from build123d import *

# Parameters (mm, degrees)
F0_W     = 70
F0_H     = 7
F1_DEPTH = 3
F2_R     = 3.49999


# Not quite as in the source:
# - a fillet or chamfer is up to 0.001 mm smaller than in the source, because OpenCascade refuses the exact size


with BuildPart() as f1:
    # F0 (on Top) → F1 (new body)
    with BuildSketch(Plane.XY):
        Rectangle(F0_W, F0_H)
        with BuildLine():
            Line((-20, -1.6), (-30, -1.6))
            ThreePointArc((-30, -1.6), (-31.6, 0), (-30, 1.6))
            Line((-30, 1.6), (-20, 1.6))
            ThreePointArc((-20, 1.6), (-18.4, 0), (-20, -1.6))
        make_face(mode=Mode.SUBTRACT)
        with BuildLine():
            Line((20, 1.6), (30, 1.6))
            ThreePointArc((30, 1.6), (31.6, 0), (30, -1.6))
            Line((30, -1.6), (20, -1.6))
            ThreePointArc((20, -1.6), (18.4, 0), (20, 1.6))
        make_face(mode=Mode.SUBTRACT)
    extrude(amount=F1_DEPTH)

    # F2 (radius 3.5 in the source; OpenCascade refuses exactly that, so slightly less here)
    f2_edges = [f1.edges().sort_by_distance(p)[0] for p in [
        (-35, 3.5, 1.5),
        (-35, -3.5, 1.5),
        (35, 3.5, 1.5),
        (35, -3.5, 1.5),
    ]]
    fillet(f2_edges, radius=F2_R)


solid = f1.part
Verification items for the finished model (mm, model axes). A direction names the side the tool comes from. Coordinates: 2 decimals unless noted, no trailing zeros. Loops run counter-clockwise (first coordinate to the right, second up) from the corner with the lowest first, then second, coordinate; pieces in that order, holes last. Notation, with made-up numbers: M 40,39.5 L 67,39.5 A33 cw 67,77.5 Z; hole C 9.25,-34.5 d8. An arc over 180 degrees is marked long. One line per item, written item: value.
1. Mould release check, pull along X, two halves, no side actions. Record for faces 3 (the cylindrical face through (-31.6, 0, 1.5)), 4 (the flat face through (0, -3.5, 1)), 5 (the flat face through (25, 1.6, 1)), 6 (the cylindrical face through (33.95, 2.5, 1.52)): pulls with the +X half, pulls with the -X half, needs draft (parallel to the pull), parting line crosses it, or undercut.
Answers follow:
face 3: undercut
face 4: needs draft
face 5: undercut
face 6: pulls with the +X half
2. Set-up check for faces 1 (the cylindrical face through (18.4, 0, 1.5)), 2 (the cylindrical face through (-34, 2.45, 1.52)): record each of +Z, -Z, +X, -X, +Y, -Y from which the full face is reachable in a straight line by a thin tool's end or side.
Answers follow:
face 1: +Z, -Z
face 2: +Z, -Z, -X, +Y
3. Material ranges on line 1 along X through (y, z) = (1, 2.5); line 2 along Y through (x, z) = (-26, 0.6); line 3 along X through (y, z) = (1.25, 0.5), recorded low to high. Write a range as from..to.
Answers follow:
line 1: -34.85..-31.25, -18.75..18.75, 31.25..34.85
line 2: -3.5..-1.6, 1.6..3.5
line 3: -34.77..-31, -19..19, 31..34.77
4. Section check B-B on y = 0.75. Record the cut outline in (x, z), plus the area to 3 significant figures.
Answers follow:
outline: M -34.92,0 L -31.41,0 L -31.41,3 L -34.92,3 Z; M -18.59,0 L 18.59,0 L 18.59,3 L -18.59,3 Z; M 31.41,0 L 34.92,0 L 34.92,3 L 31.41,3 Z
area: 133 mm^2
5. Section check A-A on z = 1.8. Give the number of separate pieces and of enclosed holes in the cut face, plus the area to 3 significant figures.
Answers follow:
separate pieces: 1
enclosed holes: 2
area: 399 mm^2
